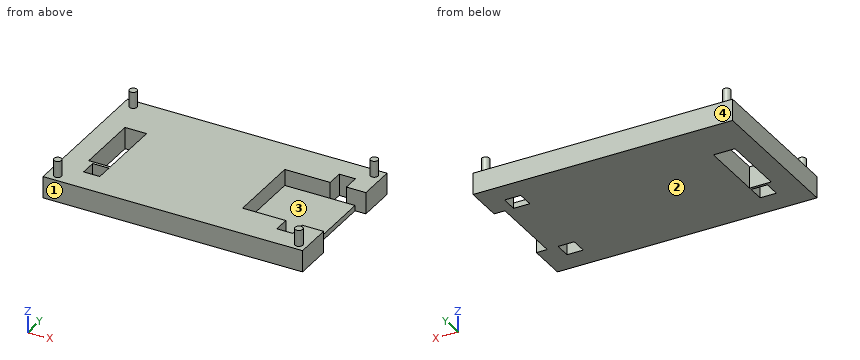
```python
from build123d import *

# Parameters (mm, degrees)
SKETCH_W               = 48
SKETCH_H               = 28
PAD_DEPTH              = 4
SKETCH001_W            = 14
SKETCH001_H            = 3
POCKET_DEPTH           = 15
SKETCH002_W            = 4
SKETCH002_H            = 12
SKETCH002_W_2          = 3
SKETCH002_H_2          = 3
POCKET001_DEPTH        = 4.001
SKETCH003_R            = 0.7
PAD001_DEPTH           = 3
FUSION_PLACEMENT_ANGLE = 180
SKETCH004_W            = 14
SKETCH004_H            = 1.055855
POCKET002_DEPTH        = 2


with BuildPart() as pocket001:
    # Sketch → Pad (new body)
    with BuildSketch(Plane.XY):
        with Locations((24, 14)):
            Rectangle(SKETCH_W, SKETCH_H)
    extrude(amount=PAD_DEPTH)

    # Sketch001 → Pocket (cut)
    with BuildSketch(Plane(origin=(0, 0, 0), x_dir=(0, -1, 0), z_dir=(-1, 0, 0))):
        with Locations((-14, 1.5)):
            Rectangle(SKETCH001_W, SKETCH001_H)
    extrude(amount=-POCKET_DEPTH, mode=Mode.SUBTRACT)

    # Sketch002 → Pocket001 (cut, through all)
    with BuildSketch(Plane.XY.offset(4)):
        with Locations((42, 14)):
            Rectangle(SKETCH002_W, SKETCH002_H)
        with Locations((41.5, 6)):
            Rectangle(SKETCH002_W_2, SKETCH002_H_2)
        with Locations((5.5, 5.5)):
            Rectangle(SKETCH002_W_2, SKETCH002_H_2)
        with Locations((5.098741, 22.5)):
            Rectangle(SKETCH002_W_2, SKETCH002_H_2)
    extrude(amount=-POCKET001_DEPTH, mode=Mode.SUBTRACT)


with BuildPart() as pocket002:
    # Pad001 base: copy of Pocket001
    add(pocket001.part)

    # Sketch003 → Pad001 (new body)
    with BuildSketch(Plane(origin=(0, 0, 0), x_dir=(1, 0, 0), z_dir=(0, 0, -1))):
        with Locations((1.5, -1.5)):
            Circle(SKETCH003_R)
        with Locations((1.5, -26.5)):
            Circle(SKETCH003_R)
        with Locations((46.109886, -26.5)):
            Circle(SKETCH003_R)
        with Locations((46.109886, -1.5)):
            Circle(SKETCH003_R)
    extrude(amount=PAD001_DEPTH)

    # Fusion: union Pocket001
    add(pocket001.part)


with BuildPart() as pocket002_1:
    # Fusion placement: moved
    add(pocket002.part.rotate(Axis((0, 0, 0), (0, 1, 0)), FUSION_PLACEMENT_ANGLE))

    # Sketch004 → Pocket002 (cut)
    with BuildSketch(Plane(origin=(0, 0, 0), x_dir=(0, -1, 0), z_dir=(1, 0, 0))):
        with Locations((-14, 3.486054)):
            Rectangle(SKETCH004_W, SKETCH004_H)
    extrude(amount=-POCKET002_DEPTH, mode=Mode.SUBTRACT)


solid = pocket002_1.part
```
The model under review builds one solid part; all positions refer to its coordinate system, in mm. Face numbers are marked on the shaded views. Round coordinates to 2 decimals unless told otherwise and drop trailing zeros. Order: outer loops, then holes, each group sorted by start corner. A loop starts at its lowest first (then second) coordinate and runs counter-clockwise, first axis right, second up.
Item 1: Draft analysis for pull direction Y (two halves, no side actions). For the marked faces 1, 2, 3 and 4, state which applies: released by +Y, released by -Y, zero draft, split by the parting line, or undercut.
Working result:
face 1: released by -Y
face 2: zero draft
face 3: undercut
face 4: released by +Y
Item 2: To check wall thickness, follow probe 1 along X at (y, z) = (16.25, -0.75); probe 2 along Y at (x, z) = (-12, -2.5); probe 3 along X at (y, z) = (23.5, -0.25). State the ranges of each line that lie inside material, in increasing order.
Working result:
probe 1: x = -48 to -44, -40 to -15
probe 2: y = 0 to 7, 21 to 28
probe 3: x = -48 to -6.6, -3.6 to 0
Item 3: Add section B-B, the plane z = -1.5. State the section outline as (x, y) points.
Working result:
outline: (-48, 0) - (0, 0) - (0, 7) - (-4, 7) - (-4, 4) - (-7, 4) - (-7, 7) - (-15, 7) - (-15, 21) - (-6.6, 21) - (-6.6, 24) - (-3.6, 24) - (-3.6, 21) - (0, 21) - (0, 28) - (-48, 28) - close; hole (-44, 8) - (-40, 8) - (-40, 20) - (-44, 20) - close; hole (-43, 4.5) - (-40, 4.5) - (-40, 7.5) - (-43, 7.5) - close
Item 4: Add section A-A, the plane x = -42. State the section outline as (y, z) points, and give its area (3 significant figures).
Working result:
outline: (0, -4) - (4.5, -4) - (4.5, 0) - (0, 0) - close; (7.5, -4) - (8, -4) - (8, 0) - (7.5, 0) - close; (20, -4) - (28, -4) - (28, 0) - (20, 0) - close
area: 52.0 mm2
Item 5: Add section C-C, the plane y = 11. State the section outline as (x, z) points.
Working result:
outline: (-48, -4) - (-44, -4) - (-44, 0) - (-48, 0) - close; (-40, -4) - (-2, -4) - (-2, -3) - (-15, -3) - (-15, 0) - (-40, 0) - close
Item 6: Add section D-D, the plane x = -1.5. State the section outline as (y, z) points, and give its area (3 significant figures).
Working result:
outline: (0, -4) - (7, -4) - (7, 0) - (2.2, 0) - (2.2, 3) - (0.8, 3) - (0.8, 0) - (0, 0) - close; (21, -4) - (28, -4) - (28, 0) - (27.2, 0) - (27.2, 3) - (25.8, 3) - (25.8, 0) - (21, 0) - close
area: 64.4 mm2
Item 7: For pin 1 (0.5 mm diameter, centred on y = 13.5, z = -3.5, fed in from +X); pin 2 (6.5 mm diameter, centred on x = -9, y = 14.5, fed in from +Z); pin 3 (6 mm diameter, centred on x = -34.5, y = 14, fed in from +Z); pin 4 (3.5 mm diameter, centred on y = 6.5, z = -1.5, fed in from +X), all flat-tipped, find the tip position at first contact; note any pin that passes through.
Working result:
pin 1: stops at x = -2
pin 2: stops at z = -3
pin 3: stops at z = 0
pin 4: stops at x = 0
